from build123d import *

# Parameters (mm, degrees)
SKETCH1_W          = 125
SKETCH1_H          = 225
BASE_FLANGE1_DEPTH = 1.3
SKETCH6_R          = 2.25
CUT_EXTRUDE1_DEPTH = 10
FILLET1_R          = 10
SKETCH7_R          = 14.5
SKETCH7_R_2        = 1.75
SKETCH7_R_3        = 2.1
SKETCH7_R_4        = 3.96875
SKETCH7_W          = 15.2
SKETCH7_H          = 8
SKETCH7_W_2        = 15.75
SKETCH7_H_2        = 13.25
CUT_EXTRUDE2_DEPTH = 10
SKETCH8_R          = 3.5
CUT_EXTRUDE3_DEPTH = 10
SKETCH9_R          = 6
CUT_EXTRUDE4_DEPTH = 10


# Sheet-metal steps are written as plain solids
with BuildPart() as part:
    # Sketch1 → Base-Flange1 (new body)
    with BuildSketch(Plane(origin=(0, 0, 0), x_dir=(1, 0, 0), z_dir=(0, 1, 0))):
        with Locations((-1.187869711, 10.618580575)):
            Rectangle(SKETCH1_W, SKETCH1_H)
    extrude(amount=-BASE_FLANGE1_DEPTH)

    # Sketch6 → Cut-Extrude1 (cut)
    with BuildSketch(Plane(origin=(0, 0, 0), x_dir=(1, 0, 0), z_dir=(0, 1, 0))):
        with Locations(Location((53.812130289, 115.618580576, 0), (0, 0, 270))):
            Circle(SKETCH6_R)
        with Locations(Location((53.812130289, -94.381419424, 0), (0, 0, 270))):
            Circle(SKETCH6_R)
        with Locations(Location((-56.187869711, -94.381419424, 0), (0, 0, 270))):
            Circle(SKETCH6_R)
        with Locations(Location((-56.187869711, 115.618580576, 0), (0, 0, 270))):
            Circle(SKETCH6_R)
        with Locations(Location((53.812130289, 10.618580576, 0), (0, 0, 270))):
            Circle(SKETCH6_R)
        with Locations(Location((-56.187869711, 10.618580576, 0), (0, 0, 270))):
            Circle(SKETCH6_R)
    extrude(amount=-CUT_EXTRUDE1_DEPTH, mode=Mode.SUBTRACT)

    # Fillet1
    fillet1_edges = [part.edges().sort_by_distance(p)[0] for p in [
        (61.312130289, -0.65, 101.881419425),
        (-63.687869711, -0.65, 101.881419425),
        (-63.687869711, -0.65, -123.118580575),
        (61.312130289, -0.65, -123.118580575),
    ]]
    fillet(fillet1_edges, radius=FILLET1_R)

    # Sketch7 → Cut-Extrude2 (cut)
    with BuildSketch(Plane(origin=(0, 0, 0), x_dir=(1, 0, 0), z_dir=(0, 1, 0))):
        with Locations(Location((22, -70, 0), (0, 0, 270))):
            Circle(SKETCH7_R)
        with Locations(Location((-22, -70, 0), (0, 0, 270))):
            Circle(SKETCH7_R)
        with Locations(Location((23.5, -30, 0), (0, 0, 270))):
            Circle(SKETCH7_R_2)
        with Locations(Location((-23.5, -30, 0), (0, 0, 270))):
            Circle(SKETCH7_R_2)
        with Locations(Location((11.3, 0, 0), (0, 0, 270))):
            Circle(SKETCH7_R_3)
        with Locations(Location((38.7, 0, 0), (0, 0, 270))):
            Circle(SKETCH7_R_3)
        with Locations(Location((-12.5, 93.118580575, 0), (0, 0, 270))):
            Circle(SKETCH7_R_4)
        with Locations(Location((-37.5, 93.118580575, 0), (0, 0, 270))):
            Circle(SKETCH7_R_4)
        with Locations(Location((-38.7, 0, 0), (0, 0, 270))):
            Circle(SKETCH7_R_3)
        with Locations(Location((-11.3, 0, 0), (0, 0, 270))):
            Circle(SKETCH7_R_3)
        with Locations(Location((37.5, 93.118580575, 0), (0, 0, 270))):
            Circle(SKETCH7_R_4)
        with Locations(Location((12.5, 93.118580575, 0), (0, 0, 270))):
            Circle(SKETCH7_R_4)
        with Locations((9.4, -30)):
            Rectangle(SKETCH7_W, SKETCH7_H)
        with Locations((-9.4, -30)):
            Rectangle(SKETCH7_W, SKETCH7_H)
        with Locations((25, 0)):
            Rectangle(SKETCH7_W_2, SKETCH7_H_2)
        with Locations((-25, 0)):
            Rectangle(SKETCH7_W_2, SKETCH7_H_2)
    extrude(amount=-CUT_EXTRUDE2_DEPTH, mode=Mode.SUBTRACT)

    # Sketch8 → Cut-Extrude3 (cut)
    with BuildSketch(Plane(origin=(0, 0, 0), x_dir=(1, 0, 0), z_dir=(0, 1, 0))):
        with Locations(Location((-37.5, 66.559290288, 0), (0, 0, 270))):
            Circle(SKETCH8_R)
        with Locations(Location((-37.5, 40, 0), (0, 0, 270))):
            Circle(SKETCH8_R)
        with Locations(Location((41.5, -30, 0), (0, 0, 270))):
            Circle(SKETCH8_R)
    extrude(amount=-CUT_EXTRUDE3_DEPTH, mode=Mode.SUBTRACT)

    # Sketch9 → Cut-Extrude4 (cut)
    with BuildSketch(Plane(origin=(0, 0, 0), x_dir=(1, 0, 0), z_dir=(0, 1, 0))):
        with Locations(Location((37.5, 40, 0), (0, 0, 270))):
            Circle(SKETCH9_R)
        with Locations(Location((37.5, 66.559290288, 0), (0, 0, 270))):
            Circle(SKETCH9_R)
        with Locations(Location((0, 66.559290288, 0), (0, 0, 270))):
            Circle(SKETCH9_R)
        with Locations(Location((0, 40, 0), (0, 0, 270))):
            Circle(SKETCH9_R)
    extrude(amount=-CUT_EXTRUDE4_DEPTH, mode=Mode.SUBTRACT)


solid = part.part
Design review of the part built by this model. Coordinates are the model's own, in mm. Coordinates: 2 decimals unless noted, no trailing zeros. Order: outer loops, then holes, each group sorted by start corner. A loop starts at its lowest first (then second) coordinate and runs counter-clockwise, first axis right, second up.
Item 1: For line 1 (X direction, y = -0.3, z = -40); line 2 (X direction, y = -0.35, z = 30); line 3 (X direction, y = -0.55, z = -9.5), list the stretches that pass through material, from the lowest coordinate up.
Item 2: Take a section at B-B, the plane x = -19.5. Write out the cut boundary in (y, z) (3 decimals).
Item 3: For pin 1 Ø23 at (x, z) = (22, 70) entering from +Y, flat-tipped, find the tip position at first contact; note if it passes through.
Item 4: Take a section at A-A, the plane z = 0. Write out the cut boundary in (x, y) (3 decimals).
Item 5: Take a section at C-C, the plane z = 70. Write out the cut boundary in (x, y), then the cut area to 3 significant figures.
Item 6: Take a section at D-D, the plane z = -92. Write out the cut boundary in (x, y).
Item 7: The part is to be moulded in two halves that separate along X. For faces 1 (the cylindrical face through (9.25, -0.64, -0.46)), 2 (the cylindrical face through (58.305, -0.659, -120.267)), 3 (the flat face through (-2, 0, -12)), say which applies: pulls with the +X half, pulls with the -X half, needs draft (parallel to the pull), parting line crosses it, or undercut.
The answers:
1. line 1: x = -63.69 to -41, -34 to -6, 6 to 31.5, 43.5 to 61.31
1. line 2: x = -63.69 to -25.25, -21.75 to -17, -1.8 to 1.8, 17 to 21.75, 25.25 to 38, 45 to 61.31
1. line 3: x = -63.69 to -58.14, -54.24 to 51.86, 55.76 to 61.31
2. outline: (-1.3, -123.119) - (0, -123.119) - (0, -6.625) - (-1.3, -6.625) - close; (-1.3, 6.625) - (0, 6.625) - (0, 55.717) - (-1.3, 55.717) - close; (-1.3, 84.283) - (0, 84.283) - (0, 101.881) - (-1.3, 101.881) - close
3. pin 1: passes through
4. outline: (-63.688, -1.3) - (-40.8, -1.3) - (-40.8, 0) - (-63.688, 0) - close; (-36.6, -1.3) - (-32.875, -1.3) - (-32.875, 0) - (-36.6, 0) - close; (-17.125, -1.3) - (-13.4, -1.3) - (-13.4, 0) - (-17.125, 0) - close; (-9.2, -1.3) - (9.2, -1.3) - (9.2, 0) - (-9.2, 0) - close; (13.4, -1.3) - (17.125, -1.3) - (17.125, 0) - (13.4, 0) - close; (32.875, -1.3) - (36.6, -1.3) - (36.6, 0) - (32.875, 0) - close; (40.8, -1.3) - (61.312, -1.3) - (61.312, 0) - (40.8, 0) - close
5. outline: (-63.69, -1.3) - (-36.5, -1.3) - (-36.5, 0) - (-63.69, 0) - close; (-7.5, -1.3) - (7.5, -1.3) - (7.5, 0) - (-7.5, 0) - close; (36.5, -1.3) - (61.31, -1.3) - (61.31, 0) - (36.5, 0) - close
5. area: 87.1 mm2
6. outline: (-63.69, -1.3) - (-41.31, -1.3) - (-41.31, 0) - (-63.69, 0) - close; (-33.69, -1.3) - (-16.31, -1.3) - (-16.31, 0) - (-33.69, 0) - close; (-8.69, -1.3) - (8.69, -1.3) - (8.69, 0) - (-8.69, 0) - close; (16.31, -1.3) - (33.69, -1.3) - (33.69, 0) - (16.31, 0) - close; (41.31, -1.3) - (61.31, -1.3) - (61.31, 0) - (41.31, 0) - close
7. face 1: undercut
7. face 2: pulls with the +X half
7. face 3: needs draft
